Here's how the part is built. I have some questions about the finished solid (model axes, mm). A direction names the side the tool comes from. Coordinates: 2 decimals unless noted, no trailing zeros. Write each loop counter-clockwise with the first axis right and the second up, starting at its lowest first coordinate (ties: lowest second). Pieces come first, ordered by that corner, then holes. Notation, with made-up numbers: (9, 28) - (15, 28) arc R23 ccw to (15, 53) - close; hole circle Ø10 at (62, 79). An arc over 180 degrees is marked (long way). Answer in a Markdown table with one row per item. Add a question column.
Item 1: Imagine slicing it at C-C (x = 44). Please give me the cut outline in (y, z), plus the area to 3 significant figures.
Item 2: We'd pull the mould along Y, two halves only. Please class faces 1 (the face through (1, 10, -51)), 2 (the face through (-43, 5, -45)), 3 (the face through (0.378, 5.601, -91.908)), 4 (the face through (0, 5, -57)): +Y half, -Y half, draft (parallel to the pull), parting line (faces both ways), or undercut.
Item 3: Imagine slicing it at D-D (x = 18). Please give me the cut outline in (y, z), plus the area to 3 significant figures.
Item 4: Imagine slicing it at B-B (z = -72.5). Please give me the cut outline in (x, y).
Item 5: Imagine slicing it at A-A (x = -25). Please give me the cut outline in (y, z), plus the area to 3 significant figures.
Item 6: If I drill on probe 1 along X at (y, z) = (0.75, -63); probe 2 along Z at (x, y) = (-41.5, 2.5); probe 3 along Z at (x, y) = (27.5, 9), over which ranges is the centre line in solid material (lowest first)? Write a range as from..to.
Item 7: Which directions (+Z, -Z, +X, -X, +Y, -Y) give clear straight access to the entire face, cutting with the end or side of a thin tool? Please do faces 5 (the face through (-30, 5, -22)), 6 (the face through (-55.5, 8, -72)), 7 (the face through (30, 5, -23)), 8 (the face through (-56, 5, -57)).
Item 8: I'm going to push flat-ended pins straight in: pin 1 (4 mm diameter, centred on x = -12.5, y = 2, fed in from +Z); pin 2 (3 mm diameter, centred on x = -38.5, y = 5.5, fed in from +Z); pin 3 (5 mm diameter, centred on y = 3.5, z = -20, fed in from -X). Where does each tip first touch, or does it pass through?
from build123d import *

# Parameters (mm, degrees)
BOSS_EXTRUDE1_DEPTH     = 10
CUT_EXTRUDE1_DEPTH      = 116.537872579
CUT_EXTRUDE1_DEPTH_BACK = 116.537872579
SKETCH2_R               = 2
SKETCH2_W               = 28.5
SKETCH2_H               = 39
SKETCH5_R               = 2
SKETCH5_R_2             = 2.75
CUT_EXTRUDE2_DEPTH      = 152.973681932


with BuildPart() as part:
    # Sketch1 → Boss-Extrude1 (new body)
    with BuildSketch(Plane(origin=(0, 0, 0), x_dir=(1, 0, 0), z_dir=(0, 1, 0))):
        Polygon((30, 0), (-30, 0), (-30, 45), (-57, 45), (-57, 100), (57, 100), (57, 45), (30, 45), align=None)
    extrude(amount=BOSS_EXTRUDE1_DEPTH)

    # Sketch2 → Cut-Extrude1 (cut, two sides: drawn at the far end of the back side and taken through both)
    with BuildSketch(Plane(origin=(0, 10, 0), x_dir=(1, 0, 0), z_dir=(0, 1, 0)).offset(-CUT_EXTRUDE1_DEPTH_BACK)):
        with Locations(Location((-52, 95, 0), (0, 0, 270))):
            Circle(SKETCH2_R)
        with Locations(Location((52, 95, 0), (0, 0, 270))):
            Circle(SKETCH2_R)
        with Locations(Location((-25, 5, 0), (0, 0, 270))):
            Circle(SKETCH2_R)
        with Locations(Location((25, 5, 0), (0, 0, 270))):
            Circle(SKETCH2_R)
        with Locations((-41.25, 72.5)):
            Rectangle(SKETCH2_W, SKETCH2_H)
        with Locations((41.25, 72.5)):
            Rectangle(SKETCH2_W, SKETCH2_H)
    extrude(amount=CUT_EXTRUDE1_DEPTH + CUT_EXTRUDE1_DEPTH_BACK, mode=Mode.SUBTRACT)

    # Sketch5 → Cut-Extrude2 (cut, through all)
    with BuildSketch(Plane(origin=(57, 0, 0), x_dir=(0, 0, -1), z_dir=(1, 0, 0))):
        with Locations(Location((55, 5, 0), (0, 0, 180))):
            Circle(SKETCH5_R)
        with Locations((90, 5)):
            Circle(SKETCH5_R)
        with Locations(Location((72.5, 5, 0), (0, 0, 180))):
            Circle(SKETCH5_R_2)
    extrude(amount=-CUT_EXTRUDE2_DEPTH, mode=Mode.SUBTRACT)


solid = part.part
Here are the results:
| question | item | result |
|---|---|---|
| 1 | outline | (0, -100) - (10, -100) - (10, -92) - (0, -92) - close; (0, -53) - (10, -53) - (10, -45) - (0, -45) - close |
| 1 | area | 160 mm2 |
| 2 | face 1 | +Y half |
| 2 | face 2 | draft |
| 2 | face 3 | undercut |
| 2 | face 4 | undercut |
| 3 | outline | (0, -100) - (10, -100) - (10, 0) - (0, 0) - close; hole circle Ø5.5 at (5, -72.5); hole circle Ø4 at (5, -90); hole circle Ø4 at (5, -55) |
| 3 | area | 951 mm2 |
| 4 | outline | (-57, 0) - (-55.5, 0) - (-55.5, 2.25) - (-57, 2.25) - close; (-57, 7.75) - (-55.5, 7.75) - (-55.5, 10) - (-57, 10) - close; (-27, 0) - (27, 0) - (27, 2.25) - (-27, 2.25) - close; (-27, 7.75) - (27, 7.75) - (27, 10) - (-27, 10) - close; (55.5, 0) - (57, 0) - (57, 2.25) - (55.5, 2.25) - close; (55.5, 7.75) - (57, 7.75) - (57, 10) - (55.5, 10) - close |
| 5 | outline | (0, -100) - (10, -100) - (10, -7) - (0, -7) - close; (0, -3) - (10, -3) - (10, 0) - (0, 0) - close; hole circle Ø5.5 at (5, -72.5); hole circle Ø4 at (5, -90); hole circle Ø4 at (5, -55) |
| 5 | area | 911 mm2 |
| 6 | probe 1 | x = -57..-55.5, -27..27, 55.5..57 |
| 6 | probe 2 | z = -100..-92, -53..-45 |
| 6 | probe 3 | z = -100..-92, -53..0 |
| 7 | face 5 | +Z, -X, +Y, -Y |
| 7 | face 6 | +Y, -Y |
| 7 | face 7 | +Z, +X, +Y, -Y |
| 7 | face 8 | +X, -X |
| 8 | pin 1 | stops at z = 0 |
| 8 | pin 2 | stops at z = -45 |
| 8 | pin 3 | stops at x = -30 |
